```python
from build123d import *

# Parameters (mm, degrees)
SKETCH_1_W      = 20
SKETCH_1_H      = 30
EXTRUDE_1_DEPTH = 20
EXTRUDE_2_DEPTH = 40
FILLET_1_R      = 10


with BuildPart() as part:
    # 草圖1 → 填料-伸長1 (new body)
    with BuildSketch(Plane(origin=(0, 0, 0), x_dir=(1, 0, 0), z_dir=(0, 1, 0))):
        with Locations((10, 15)):
            Rectangle(SKETCH_1_W, SKETCH_1_H)
    extrude(amount=EXTRUDE_1_DEPTH)

    # 草圖1<3> → 填料-伸長2 (add)
    with BuildSketch(Plane(origin=(0, 0, 0), x_dir=(1, 0, 0), z_dir=(0, 1, 0))):
        Polygon((0, 50), (0, 30), (20, 30), (40, 30), (40, 50), align=None)
    extrude(amount=EXTRUDE_2_DEPTH)

    # 圓角1
    fillet_1_edges = [part.edges().sort_by_distance(p)[0] for p in [
        (10, 20, 0),
        (10, 20, -30),
        (40, 40, -40),
    ]]
    fillet(fillet_1_edges, radius=FILLET_1_R)


solid = part.part
```
For this review, take the finished solid that the model builds, in its own axes (mm). A direction names the side the tool comes from. Coordinates: 2 decimals unless noted, no trailing zeros. Write each loop counter-clockwise with the first axis right and the second up, starting at its lowest first coordinate (ties: lowest second). Pieces come first, ordered by that corner, then holes.
(1) Add section D-D on y = 19. Give the boundary of the cut face in (x, z), then the cut area to 3 significant figures.
(2) Add section C-C on y = 28. Give the boundary of the cut face in (x, z), then the cut area to 3 significant figures.
(3) Add section A-A on x = 10.5. Give the boundary of the cut face in (y, z).
(4) Wall thickness on probe 1 along Z at (x, y) = (36.5, 19); probe 2 along Y at (x, z) = (16, -15): over which ranges is each line inside the solid? List them lowest first.
(5) For pin 1 Ø1.5 at (y, z) = (9, -14.5) entering from +X; pin 2 Ø3 at (x, y) = (16, 17) entering from +Z; pin 3 Ø1 at (x, y) = (34.5, 36) entering from +Z; pin 4 Ø8 at (y, z) = (24, -36) entering from -X, all flat-tipped, find the tip position at first contact; note any pin that passes through.
(6) Add section B-B on z = -17. Give the boundary of the cut face in (x, y).
(7) Tool access review of faces 1 (the face through (24, 24, -30)), 2 (the face through (10, 5, 0)), 3 (the face through (10, 20, -15)), 4 (the face through (20, 11, -15)): name each direction out of +Z, -Z, +X, -X, +Y, -Y from which nothing blocks a thin tool from reaching the whole face with its end or side.
Answer sheet:
1. outline: (0, -50) - (40, -50) - (40, -30) - (20, -30) - (20, -5.64) - (0, -5.64) - close
1. area: 1,290 mm2
2. outline: (0, -50) - (40, -50) - (40, -30) - (20, -30) - (20, -29.8) - (0, -29.8) - close
2. area: 804 mm2
3. outline: (0, -50) - (40, -50) - (40, -30) - (30, -30) arc R10 cw to (20, -20) - (20, -10) arc R10 ccw to (10, 0) - (0, 0) - close
4. probe 1: z = -50 to -30
4. probe 2: y = 0 to 20
5. pin 1: stops at x = 20
5. pin 2: stops at z = -1.65
5. pin 3: stops at z = -30
5. pin 4: stops at x = 0
6. outline: (0, 0) - (20, 0) - (20, 20) - (0, 20) - close
7. face 1: +Z, +X, +Y
7. face 2: +Z, +X, -X, +Y, -Y
7. face 3: +Z, +X, -X, +Y
7. face 4: +Z, +X, +Y, -Y
